Read the model definition and answer for the solid it produces. Units are mm, in the model's axes. Give positions to 0.01 mm unless a question says otherwise; leave off trailing zeros. Write each loop counter-clockwise with the first axis right and the second up, starting at its lowest first coordinate (ties: lowest second). Pieces come first, ordered by that corner, then holes. Notation, with made-up numbers: (76, -30) - (94, -30) arc R19 cw to (94, -23) - close; hole circle Ø5 at (57.25, 74). An arc over 180 degrees is marked (long way). Use CSV: the item, a comma, the result in double quotes. Start each with the question number.
from build123d import *

# Parameters (mm, degrees)
SKETCH1_W             = 30
SKETCH1_H             = 30
BOSS_EXTRUDE1_DEPTH   = 10
SKETCH2_W             = 30
SKETCH2_H             = 30
SKETCH2_W_2           = 20
SKETCH2_H_2           = 20
BOSS_EXTRUDE2_DEPTH   = 10
SKETCH2_W_3           = 5
SKETCH2_H_3           = 3.748828889
BOSS_EXTRUDE2_2_DEPTH = 10
BOSS_EXTRUDE2_3_DEPTH = 10
SKETCH3_W             = 30
SKETCH3_H             = 30
BOSS_EXTRUDE3_DEPTH   = 10
SKETCH4_R             = 3.1
CUT_EXTRUDE1_DEPTH    = 10
SKETCH5_R             = 3.1
CUT_EXTRUDE2_DEPTH    = 10
CUT_EXTRUDE3_START    = -30
SKETCH8_R             = 1
CUT_EXTRUDE3_DEPTH    = 30


with BuildPart() as part:
    # Sketch1 → Boss-Extrude1 (new body)
    with BuildSketch(Plane.XY):
        Rectangle(SKETCH1_W, SKETCH1_H)
    extrude(amount=BOSS_EXTRUDE1_DEPTH)

    # Sketch5 → Cut-Extrude2 (cut)
    with BuildSketch(Plane(origin=(0, 0, 0), x_dir=(-1, 0, 0), z_dir=(0, 0, -1))):
        with Locations((-6, -0.372899474)):
            Circle(SKETCH5_R)
    extrude(amount=-CUT_EXTRUDE2_DEPTH, mode=Mode.SUBTRACT)


with BuildPart() as body_2:
    # Sketch2 → Boss-Extrude2 (new body)
    with BuildSketch(Plane.XY.offset(10)):
        Rectangle(SKETCH2_W, SKETCH2_H)
        Rectangle(SKETCH2_W_2, SKETCH2_H_2, mode=Mode.SUBTRACT)
    extrude(amount=BOSS_EXTRUDE2_DEPTH)


with BuildPart() as body_3:
    # Sketch2 → Boss-Extrude2 2 (new body)
    with BuildSketch(Plane.XY.offset(10)):
        with Locations((0, 5.374414445)):
            Rectangle(SKETCH2_W_3, SKETCH2_H_3)
    extrude(amount=BOSS_EXTRUDE2_2_DEPTH)


with BuildPart() as body_4:
    # Sketch2 → Boss-Extrude2 3 (new body)
    with BuildSketch(Plane.XY.offset(10)):
        with Locations((0, -5.374414445)):
            Rectangle(SKETCH2_W_3, SKETCH2_H_3)
    extrude(amount=BOSS_EXTRUDE2_3_DEPTH)


with BuildPart() as body_5:
    # Sketch3 → Boss-Extrude3 (new body)
    with BuildSketch(Plane.XY.offset(20)):
        Rectangle(SKETCH3_W, SKETCH3_H)
    extrude(amount=BOSS_EXTRUDE3_DEPTH)

    # Sketch4 → Cut-Extrude1 (cut)
    with BuildSketch(Plane.XY.offset(30)):
        with Locations((-6, 0)):
            Circle(SKETCH4_R)
    extrude(amount=-CUT_EXTRUDE1_DEPTH, mode=Mode.SUBTRACT)


with BuildPart() as cut_extrude3_tool:
    # Sketch8 → Cut-Extrude3 (new body)
    with BuildSketch(Plane.XY.offset(30).offset(CUT_EXTRUDE3_START)):
        with Locations((-12, -12)):
            Circle(SKETCH8_R)
        with Locations((12.878679656, 12.878679656)):
            Circle(SKETCH8_R)
    extrude(amount=CUT_EXTRUDE3_DEPTH)


with BuildPart() as part_1:
    add(part.part)

    # Cut-Extrude3: cut by cut_extrude3_tool
    add(cut_extrude3_tool.part, mode=Mode.SUBTRACT)


with BuildPart() as body_2_1:
    add(body_2.part)

    # Cut-Extrude3: cut by cut_extrude3_tool
    add(cut_extrude3_tool.part, mode=Mode.SUBTRACT)


with BuildPart() as body_5_1:
    add(body_5.part)

    # Cut-Extrude3: cut by cut_extrude3_tool
    add(cut_extrude3_tool.part, mode=Mode.SUBTRACT)


solid = body_5_1.part
(1) The part is cut by section B-B on y = 0. Write down the section's boundary in (x, z), plus the area to 3 significant figures.
(2) For a pull along X with two mould halves and no side action, classify faces 1 (the face through (-9.1, 0.1, 25.1)), 2 (the face through (0, 15, 25)), 3 (the face through (15, 0, 25)), 4 (the face through (-15, 0, 25)) as pulls with the +X half, pulls with the -X half, needs draft (parallel to the pull), parting line crosses it, or undercut.
(3) The part is cut by section C-C on z = 26.5. Write down the section's boundary in (x, y), plus the area to 3 significant figures.
(4) Consider probe 1 along Y at (x, z) = (-6, 27.5); probe 2 along Y at (x, z) = (-11.75, 28.75); probe 3 along X at (y, z) = (13.5, 28). Determine where each line is inside the solid, lowest interval first.
(5) The part is cut by section A-A on x = -6. Write down the section's boundary in (y, z), plus the area to 3 significant figures.
Reported:
1,outline,"(-15, 20) - (-9.1, 20) - (-9.1, 30) - (-15, 30) - close; (-2.9, 20) - (15, 20) - (15, 30) - (-2.9, 30) - close"
1,area,"238 mm²"
2,face 1,"undercut"
2,face 2,"needs draft"
2,face 3,"pulls with the +X half"
2,face 4,"pulls with the -X half"
3,outline,"(-15, -15) - (15, -15) - (15, 15) - (-15, 15) - close; hole circle Ø2 at (-12, -12); hole circle Ø6.2 at (-6, 0); hole circle Ø2 at (12.88, 12.88)"
3,area,"864 mm²"
4,probe 1,"-15 to -3.1, 3.1 to 15"
4,probe 2,"-15 to -12.97, -11.03 to 15"
4,probe 3,"-15 to 12.1, 13.66 to 15"
5,outline,"(-15, 20) - (-3.1, 20) - (-3.1, 30) - (-15, 30) - close; (3.1, 20) - (15, 20) - (15, 30) - (3.1, 30) - close"
5,area,"238 mm²"
